from build123d import *

# Parameters (mm, degrees)
F0_W      = 87.133936584
F0_H      = 95.9787741303
F1_DEPTH  = 46.1022332311
F2_W      = 51.2357354164
F2_H      = 64.0120953321
F3_DEPTH  = 79.969028011
F6_R      = 10.6062460881
F7_DEPTH  = 56.2525093555
F8_W      = 38.8421155512
F8_H      = 9.6180737019
F9_DEPTH  = 59.3906808645
F10_W     = 51.2357354164
F10_H     = 13.8573199511
F10_W_2   = 11.7768868804
F10_W_3   = 12.2887119651
F11_DEPTH = 13.6597724631
F12_R     = 20
F13_SIZE  = 5.08


# Not quite as in the source:
# - a feature names something its author has since deleted; it is built from what else it names
# - the program builds the solid bodies; features that only make, move or delete a surface that nothing else refers to are left out


with BuildPart() as f1:
    # F0 (on Front) → F1 (new body)
    with BuildSketch(Plane.XZ):
        with Locations((-0.1830421388, 6.0982592404)):
            Rectangle(F0_W, F0_H)
    extrude(amount=F1_DEPTH)

    # F2 (on face) → F3 (cut)
    with BuildSketch(Plane.XZ.offset(46.1022332311)):
        with Locations((0.2559125423, 5.0961896777)):
            Rectangle(F2_W, F2_H)
    extrude(amount=-F3_DEPTH, mode=Mode.SUBTRACT)

    # F6 (on Right) → F7 (join, symmetric)
    with BuildSketch(Plane.YZ):
        with Locations((-23.2529193163, 0)):
            Circle(F6_R)
    extrude(amount=F7_DEPTH, both=True)

    # F8 (on face) → F9 (cut)
    with BuildSketch(Plane(origin=(0, 0, 0), x_dir=(-1, 0, 0), z_dir=(0, 1, 0))):
        with Locations((0, 46.3703721762)):
            Rectangle(F8_W, F8_H)
    extrude(amount=-F9_DEPTH, mode=Mode.SUBTRACT)

    # F10 (on face) → F11 (join, symmetric)
    with BuildSketch(Plane.XZ.offset(46.1022332311)):
        with Locations((0.2559125423, 0)):
            Rectangle(F10_W, F10_H)
        with Locations((31.7622236907, 0)):
            Rectangle(F10_W_2, F10_H)
        with Locations((-31.5063111484, 0)):
            Rectangle(F10_W_3, F10_H)
    extrude(amount=F11_DEPTH, both=True)

    # F12
    f12_edges = [f1.edges().sort_by_distance(p)[0] for p in [
        (-43.75001, -23.051117, 54.087646),
        (43.383926, -23.051117, 54.087646),
    ]]
    fillet(f12_edges, radius=F12_R)

    # F13
    f13_edges = [f1.edges().sort_by_distance(p)[0] for p in [
        (0, -59.762006, 6.92866),
    ]]
    chamfer(f13_edges, length=F13_SIZE)


solid = f1.part
For this review, take the finished solid that the model builds, in its own axes (mm). A direction names the side the tool comes from. Round coordinates to 2 decimals unless told otherwise and drop trailing zeros. Write each loop counter-clockwise with the first axis right and the second up, starting at its lowest first coordinate (ties: lowest second). Pieces come first, ordered by that corner, then holes. Notation, with made-up numbers: (61, -19.75) - (111, -19.75) arc R24 cw to (111, 0.25) - close; hole circle Ø11 at (64.5, 77). An arc over 180 degrees is marked (long way). Use a Markdown table: item, result.
Q1. Wall thickness on line 1 along Z through (x, y) = (-15, -39); line 2 along Z through (x, y) = (17, -11); line 3 along Z through (x, y) = (-22, -40): over which ranges is each line inside the solid? List them lowest first.
Derived:
| item | result |
|---|---|
| line 1 | z = -41.89 to -26.91, -6.93 to 6.93, 37.1 to 41.56, 51.18 to 54.09 |
| line 2 | z = -41.89 to -26.91, 37.1 to 41.56, 51.18 to 54.09 |
| line 3 | z = -41.89 to -26.91, -6.93 to 6.93, 37.1 to 54.09 |
Q2. We need section C-C (z = 24.5). Give the boundary of the cut face in (x, y).
Derived:
| item | result |
|---|---|
| outline | (-43.75, -46.1) - (-25.36, -46.1) - (-25.36, 0) - (-43.75, 0) - close; (25.87, -46.1) - (43.38, -46.1) - (43.38, 0) - (25.87, 0) - close |
Q3. We need section B-B (x = 18). Give the boundary of the cut face in (y, z), plus the area to 3 significant figures.
Derived:
| item | result |
|---|---|
| outline | (-59.76, -6.93) - (-32.44, -6.93) - (-32.44, -5.3) arc R10.61 ccw (long way) to (-32.44, 5.3) - (-32.44, 6.93) - (-54.68, 6.93) - (-59.76, 1.85) - close; (-46.1, -41.89) - (0, -41.89) - (0, -26.91) - (-46.1, -26.91) - close; (-46.1, 37.1) - (0, 37.1) - (0, 41.56) - (-46.1, 41.56) - close; (-46.1, 51.18) - (0, 51.18) - (0, 54.09) - (-46.1, 54.09) - close |
| area | 1,740 mm2 |
Q4. Machinability: for faces 1 (the flat face through (0, -23, 51.179)), 2 (the flat face through (37.651, -53, 0)), 3 (the flat face through (1, -44, 6.929)), which of the approach directions +Z, -Z, +X, -X, +Y, -Y give a long, thin tool a straight path to every point of the face, cutting with its end or side? Answer none if there is none.
Derived:
| item | result |
|---|---|
| face 1 | +Y, -Y |
| face 2 | +Z, -Z, +X, -Y |
| face 3 | -Y |
Q5. We need section A-A (y = -40). Give the boundary of the cut face in (x, z), plus the area to 3 significant figures.
Derived:
| item | result |
|---|---|
| outline | (-43.75, -41.89) - (43.38, -41.89) - (43.38, 34.09) arc R20 ccw to (23.38, 54.09) - (-23.75, 54.09) arc R20 ccw to (-43.75, 34.09) - close; hole (-25.36, -26.91) - (25.87, -26.91) - (25.87, -6.93) - (-25.36, -6.93) - close; hole (-25.36, 6.93) - (25.87, 6.93) - (25.87, 37.1) - (-25.36, 37.1) - close; hole (-19.42, 41.56) - (19.42, 41.56) - (19.42, 51.18) - (-19.42, 51.18) - close |
| area | 5,250 mm2 |
Q6. Clearance check with flat-ended pins moving along their axes: pin 1 (23 mm diameter, centred on y = -13, z = 21, fed in from +X); pin 2 (3 mm diameter, centred on x = -39, z = 37, fed in from -Y); pin 3 (15 mm diameter, centred on y = -50.5, z = -1, fed in from -X). State where each tip first meets the part, or that it passes through.
Derived:
| item | result |
|---|---|
| pin 1 | stops at x = 43.38 |
| pin 2 | stops at y = -46.1 |
| pin 3 | stops at x = -43.75 |
Q7. We need section D-D (z = 0). Give the boundary of the cut face in (x, y).
Derived:
| item | result |
|---|---|
| outline | (-56.25, -33.86) - (-43.75, -33.86) - (-43.75, -46.1) - (-37.65, -46.1) - (-37.65, -59.76) - (37.65, -59.76) - (37.65, -46.1) - (43.38, -46.1) - (43.38, -33.86) - (56.25, -33.86) - (56.25, -12.65) - (43.38, -12.65) - (43.38, 0) - (25.87, 0) - (25.87, -12.65) - (-25.36, -12.65) - (-25.36, 0) - (-43.75, 0) - (-43.75, -12.65) - (-56.25, -12.65) - close |
Q8. The part is to be moulded in two halves that separate along X. For faces 4 (the flat face through (-56.253, -23, 0)), 5 (the flat face through (-1, -23, -41.891)), 6 (the flat face through (19.421, -23, 46)), say which applies: pulls with the +X half, pulls with the -X half, needs draft (parallel to the pull), parting line crosses it, or undercut.
Derived:
| item | result |
|---|---|
| face 4 | pulls with the -X half |
| face 5 | needs draft |
| face 6 | undercut |
